from build123d import *

# Parameters (mm, degrees)
BOSS_EXTRUDE1_DEPTH = 1.016
SKETCH2_W           = 1.6256
SKETCH2_H           = 1.016
BOSS_EXTRUDE2_DEPTH = 2.286


with BuildPart() as part:
    # Sketch1 → Boss-Extrude1 (new body)
    with BuildSketch(Plane(origin=(0, 0, 0), x_dir=(1, 0, 0), z_dir=(0, 1, 0))):
        with BuildLine():
            Line((0.8128, -9.8806), (-0.8128, -9.8806))
            Line((-0.8128, -9.8806), (-0.8128, -9.082302688))
            ThreePointArc((-0.8128, -9.082302688), (0, 9.1186), (0.8128, -9.082302688))
            Line((0.8128, -9.082302688), (0.8128, -9.8806))
        make_face()
        with BuildLine():
            Line((0.8128, -6.297765966), (0.8128, -5.588))
            Line((0.8128, -5.588), (-0.8128, -5.588))
            Line((-0.8128, -5.588), (-0.8128, -6.297765966))
            ThreePointArc((-0.8128, -6.297765966), (0, 6.35), (0.8128, -6.297765966))
        make_face(mode=Mode.SUBTRACT)
    extrude(amount=BOSS_EXTRUDE1_DEPTH)

    # Sketch2 → Boss-Extrude2 (add)
    with BuildSketch(Plane(origin=(0, 1.016, 0), x_dir=(1, 0, 0), z_dir=(0, 1, 0))):
        with Locations((0, -9.3726)):
            Rectangle(SKETCH2_W, SKETCH2_H)
    extrude(amount=BOSS_EXTRUDE2_DEPTH)


solid = part.part
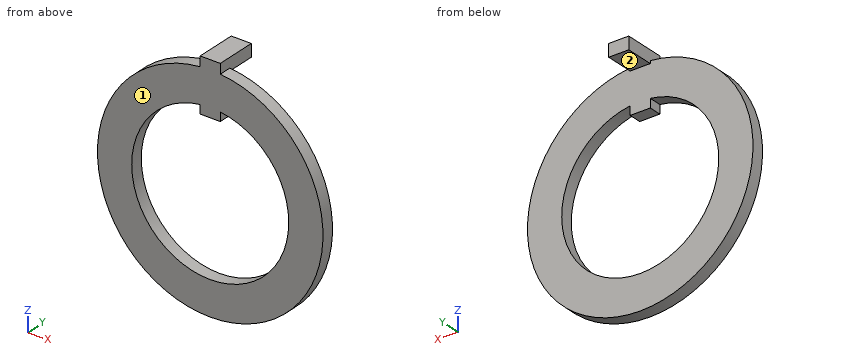
CAD build for the part. Positions are in the model's coordinates, mm. Face numbers are marked on the shaded views. A direction names the side the tool comes from. Give positions to 0.01 mm unless a question says otherwise; leave off trailing zeros. Write each loop counter-clockwise with the first axis right and the second up, starting at its lowest first coordinate (ties: lowest second). Pieces come first, ordered by that corner, then holes. Notation, with made-up numbers: (68.25, -17) -> (117.25, -17) arc R28 ccw to (117.25, 15) -> close; hole circle Ø9 at (50.5, -4.75). An arc over 180 degrees is marked (long way). Return JSON: item names as keys, results as strings.
Item 1: Drill centre lines: probe 1 along X at (y, z) = (0.25, 0); probe 2 along Y at (x, z) = (-6.75, -2.5); probe 3 along Z at (x, y) = (0, 2.1). Where is each one in solid material? Low to high.
Answer below:
{"probe 1": "x = -9.12 to -6.35, 6.35 to 9.12", "probe 2": "y = 0 to 1.02", "probe 3": "z = 8.86 to 9.88"}
Item 2: Drop flat-ended pins along their axis: pin 1 (0.8 mm diameter, centred on y = 2, z = 9.5, fed in from -X); pin 2 (1.5 mm diameter, centred on x = -4.5, z = 5, fed in from +Y); pin 3 (0.5 mm diameter, centred on x = 0, y = 2, fed in from -Z). Give the stop position or say it passes through.
Answer below:
{"pin 1": "stops at x = -0.81", "pin 2": "stops at y = 1.02", "pin 3": "stops at z = 8.86"}
Item 3: Band-saw the part on D-D (z = 5). List the corners of the cut face in (x, y).
Answer below:
{"outline": "(-7.63, 0) -> (-3.91, 0) -> (-3.91, 1.02) -> (-7.63, 1.02) -> close; (3.91, 0) -> (7.63, 0) -> (7.63, 1.02) -> (3.91, 1.02) -> close"}
Item 4: Tool access for the marked faces 1 and 2: list every direction of +Z, -Z, +X, -X, +Y, -Y with a clear straight run to the whole face (end or side of a thin tool).
Answer below:
{"face 1": "+Z, -Z, +X, -X, -Y", "face 2": "-Z, +X, -X, +Y"}
Item 5: Band-saw the part on C-C (y = 0.65). List the corners of the cut face in (x, z), then the cut area to 3 significant figures.
Answer below:
{"outline": "(-0.81, 9.08) arc R9.12 ccw (long way) to (0.81, 9.08) -> (0.81, 9.88) -> (-0.81, 9.88) -> close; hole (-0.81, 5.59) -> (-0.81, 6.3) arc R6.35 ccw (long way) to (0.81, 6.3) -> (0.81, 5.59) -> close", "area": "137 mm2"}
Item 6: Band-saw the part on A-A (x = 0). List the corners of the cut face in (y, z), then the cut area to 3 significant figures.
Answer below:
{"outline": "(0, -9.12) -> (1.02, -9.12) -> (1.02, -6.35) -> (0, -6.35) -> close; (0, 5.59) -> (1.02, 5.59) -> (1.02, 8.86) -> (3.3, 8.86) -> (3.3, 9.88) -> (0, 9.88) -> close", "area": "9.50 mm2"}
Item 7: Band-saw the part on B-B (z = 0). List the corners of the cut face in (x, y).
Answer below:
{"outline": "(-9.12, 0) -> (-6.35, 0) -> (-6.35, 1.02) -> (-9.12, 1.02) -> close; (6.35, 0) -> (9.12, 0) -> (9.12, 1.02) -> (6.35, 1.02) -> close"}
